Geometry: final body of the model. Coordinates: model frame, mm. Give positions to 0.01 mm unless a question says otherwise; leave off trailing zeros. Return JSON: item names as keys, results as strings.
from build123d import *

# Parameters (mm, degrees)
EXTRUDE_1_DEPTH = 100


with BuildPart() as part:
    # Эскиз1 → Бобышка-Вытянуть1 (new body)
    with BuildSketch(Plane.XY):
        Polygon((-52.5, 0), (-51, 1.5), (-49, 1.5), (-47.5, 0), (-2.5, 0), (-1, 1.5), (1, 1.5), (2.5, 0), (47.5, 0), (49, 1.5), (51, 1.5), (52.5, 0), (97.5, 0), (99, 1.5), (101, 1.5), (102.5, 0), (124, 0), (125, 1), (125, 19), (124, 20), (117.55, 20), (116.55, 19), (116.55, 15), (119.75, 15), (119.75, 8), (105.25, 8), (105.25, 15), (108.45, 15), (108.45, 19), (107.45, 20), (92.55, 20), (91.55, 19), (91.55, 15), (94.75, 15), (94.75, 8), (80.25, 8), (80.25, 15), (83.45, 15), (83.45, 19), (82.45, 20), (67.55, 20), (66.55, 19), (66.55, 15), (69.75, 15), (69.75, 8), (55.25, 8), (55.25, 15), (58.45, 15), (58.45, 19), (57.45, 20), (42.55, 20), (41.55, 19), (41.55, 15), (44.75, 15), (44.75, 8), (30.25, 8), (30.25, 15), (33.45, 15), (33.45, 19), (32.45, 20), (17.55, 20), (16.55, 19), (16.55, 15), (19.75, 15), (19.75, 8), (5.25, 8), (5.25, 15), (8.45, 15), (8.45, 19), (7.45, 20), (-7.45, 20), (-8.45, 19), (-8.45, 15), (-5.25, 15), (-5.25, 8), (-19.75, 8), (-19.75, 15), (-16.55, 15), (-16.55, 19), (-17.55, 20), (-32.45, 20), (-33.45, 19), (-33.45, 15), (-30.25, 15), (-30.25, 8), (-44.75, 8), (-44.75, 15), (-41.55, 15), (-41.55, 19), (-42.55, 20), (-57.45, 20), (-58.45, 19), (-58.45, 15), (-55.25, 15), (-55.25, 8), (-69.75, 8), (-69.75, 15), (-66.55, 15), (-66.55, 19), (-67.55, 20), (-82.45, 20), (-83.45, 19), (-83.45, 15), (-80.25, 15), (-80.25, 8), (-94.75, 8), (-94.75, 15), (-91.55, 15), (-91.55, 19), (-92.55, 20), (-107.45, 20), (-108.45, 19), (-108.45, 15), (-105.25, 15), (-105.25, 8), (-119.75, 8), (-119.75, 15), (-116.55, 15), (-116.55, 19), (-117.55, 20), (-124, 20), (-125, 19), (-125, 1), (-124, 0), (-102.5, 0), (-101, 1.5), (-99, 1.5), (-97.5, 0), align=None)
    extrude(amount=-EXTRUDE_1_DEPTH)


solid = part.part
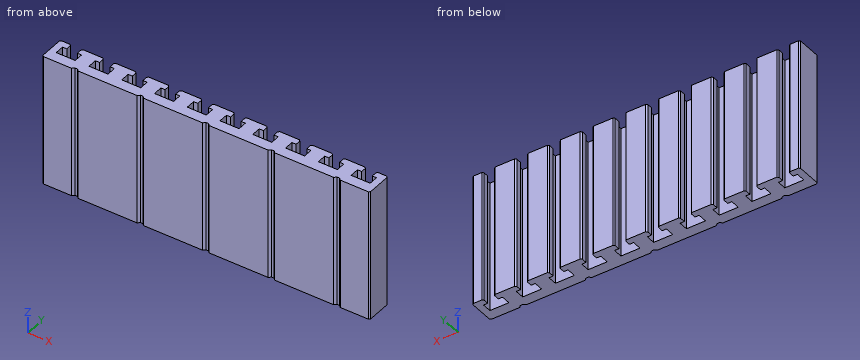
Q1. Section query A-A, the plane y = 11.25. Count the separate pieces of the cut face and the enclosed holes in it, plus the area to 3 significant figures.
Answer key:
{"separate pieces": "11", "enclosed holes": "0", "area": "10,500 mm^2"}
Q2. Pin query (flat end, axial travel): P1, Ø1.6, axis at x = -100, z = -36.5, coming from the -Y side; P2, Ø2, axis at x = 0.5, z = -58, coming from the -Y side. Return the tip coordinate at first contact, or that it passes through.
Answer key:
{"P1": "stops at y = 1.5", "P2": "stops at y = 1"}
Q3. Material intervals for probe 1 along Y at (x, z) = (44, -17); probe 2 along Y at (x, z) = (-110.5, -34.5); probe 3 along Y at (x, z) = (99, -35.5), sorted ascending. Write a range as [from, to].
Answer key:
{"probe 1": "y = [0, 8], [15, 20]", "probe 2": "y = [0, 8]", "probe 3": "y = [1.5, 20]"}
